```python
from build123d import *

# Parameters (mm, degrees)
PAD005_DEPTH    = 12
SKETCH025_R     = 2.5
POCKET019_DEPTH = 10
POCKET020_DEPTH = 1
SKETCH027_W     = 8
SKETCH027_H     = 8.3
POCKET021_DEPTH = 5
PAD006_DEPTH    = 3.5
SKETCH029_W     = 12.5
SKETCH029_H     = 5
POCKET022_DEPTH = 2


with BuildPart() as part:
    # Sketch024 → Pad005 (new body)
    with BuildSketch(Plane.XY):
        with BuildLine():
            ThreePointArc((0, 0), (0.0125001507, 3.6000868045), (0.05, 7.2))
            Line((0.05, 7.2), (0.75, 22.55))
            add(Edge.make_bspline(
                [(0.75, 22.55), (0.790433, 24.50555), (2.8995135699, 28.3383927733), (10.6468681476, 35.231617337), (14.5053016695, 34.8194742751), (20.1, 35.5)],
                knots=[0, 0, 0, 0, 0.3333333333, 0.6666666667, 1, 1, 1, 1], degree=3))
            Line((20.1, 35.5), (64.2, 35.5))
            add(Edge.make_bspline(
                [(92, 0), (92.391037, 11.810127), (88.126587, 35.076866), (64.2, 35.5)],
                knots=[0, 0, 0, 0, 1, 1, 1, 1], degree=3))
            Line((92, 0), (0, 0))
        make_face()
    extrude(amount=PAD005_DEPTH)

    # Sketch025 (on Face8 of Pad005) → Pocket019 (cut)
    with BuildSketch(Plane.XY.offset(12)):
        with Locations((17, 25)):
            Circle(SKETCH025_R)
        with BuildLine():
            ThreePointArc((84.5, 0), (82, 2.5), (79.5, 0))
            Line((79.5, 0), (84.5, 0))
        make_face()
        with BuildLine():
            Line((2, 0), (2.5758571429, 18.6857169977))
            ThreePointArc((7.6817324497, 29.5040514173), (4.0036624605, 24.625907301), (2.5758571429, 18.6857169977))
            ThreePointArc((11, 28), (9.8256709089, 29.8216112511), (7.6817324497, 29.5040514173))
            Line((11, 25), (11, 28))
            ThreePointArc((11, 25), (17, 19), (23, 25))
            Line((23, 25), (23, 31.5))
            ThreePointArc((25, 33.5), (23.5857864376, 32.9142135624), (23, 31.5))
            Line((25.1, 33.5), (25, 33.5))
            ThreePointArc((27.1, 31.5), (26.5142135624, 32.9142135624), (25.1, 33.5))
            Line((27.1, 12), (27.1, 31.5))
            ThreePointArc((27.1, 12), (27.6857864376, 10.5857864376), (29.1, 10))
            Line((31.1, 10), (29.1, 10))
            ThreePointArc((31.1, 10), (32.5142135624, 10.5857864376), (33.1, 12))
            Line((33.1, 31.5), (33.1, 12))
            ThreePointArc((35.1, 33.5), (33.6857864376, 32.9142135624), (33.1, 31.5))
            Line((49.3, 33.5), (35.1, 33.5))
            ThreePointArc((51.3, 31.5), (50.7142135624, 32.9142135624), (49.3, 33.5))
            Line((51.3, 12), (51.3, 31.5))
            ThreePointArc((51.3, 12), (51.8857864376, 10.5857864376), (53.3, 10))
            Line((55.3, 10), (53.3, 10))
            ThreePointArc((55.3, 10), (56.7142135624, 10.5857864376), (57.3, 12))
            Line((57.3, 31.4999999999), (57.3, 12))
            ThreePointArc((59.3, 33.4999999999), (57.8857864376, 32.9142135623), (57.3, 31.4999999999))
            Line((59.3, 33.5), (64.2, 33.5))
            ThreePointArc((87.491325765, 7.8139309331), (81.5019467421, 25.7859071373), (64.2, 33.5))
            ThreePointArc((85.5, 6), (86.8468225322, 6.521463877), (87.491325765, 7.8139309331))
            Line((82, 6), (85.5, 6))
            ThreePointArc((82, 6), (77.7573593129, 4.2426406871), (76, 0))
            Line((22, 0), (76, 0))
            Line((22, 1), (22, 0))
            Line((16, 1), (22, 1))
            Line((16, 0), (16, 1))
            Line((2, 0), (16, 0))
        make_face()
    extrude(amount=-POCKET019_DEPTH, mode=Mode.SUBTRACT)

    # Sketch026 (on Face3 of Pocket019) → Pocket020 (cut)
    with BuildSketch(Plane.XZ):
        Polygon((22, 12), (22, 4), (18, 10), (16, 10), (16, 12), align=None)
    extrude(amount=-POCKET020_DEPTH, mode=Mode.SUBTRACT)

    # Sketch027 → Pocket021 (cut)
    with BuildSketch(Plane.YZ):
        with Locations((4, 6.15)):
            Rectangle(SKETCH027_W, SKETCH027_H)
    extrude(amount=POCKET021_DEPTH, mode=Mode.SUBTRACT)

    # Sketch028 (on Face8 of Pocket021) → Pad006 (join)
    with BuildSketch(Plane.XY.offset(12)):
        with BuildLine():
            ThreePointArc((31.1, 10), (32.5142135624, 10.5857864376), (33.1, 12))
            Line((33.1, 12), (33.1, 14))
            ThreePointArc((33.1, 14), (32.5142135624, 15.4142135624), (31.1, 16))
            Line((29.1, 16), (31.1, 16))
            ThreePointArc((29.1, 16), (27.6857864376, 15.4142135624), (27.1, 14))
            Line((27.1, 12), (27.1, 14))
            ThreePointArc((27.1, 12), (27.6857864376, 10.5857864376), (29.1, 10))
            Line((29.1, 10), (31.1, 10))
        make_face()
        with BuildLine():
            ThreePointArc((51.3, 12), (51.8857864376, 10.5857864376), (53.3, 10))
            Line((53.3, 10), (55.3, 10))
            ThreePointArc((55.3, 10), (56.7142135624, 10.5857864376), (57.3, 12))
            Line((57.3, 12), (57.3, 14))
            ThreePointArc((57.3, 14), (56.7142135624, 15.4142135624), (55.3, 16))
            Line((53.3, 16), (55.3, 16))
            ThreePointArc((53.3, 16), (51.8857864376, 15.4142135624), (51.3, 14))
            Line((51.3, 12), (51.3, 14))
        make_face()
    extrude(amount=PAD006_DEPTH)

    # Mirrored002: part across XZ


with BuildPart() as part_1:
    add(part.part)
    add(part.part.mirror(Plane.XZ))

    # Sketch029 (on Face33 of Mirrored002) → Pocket022 (cut)
    with BuildSketch(Plane(origin=(0, 35.5, 0), x_dir=(-1, 0, 0), z_dir=(0, 1, 0))):
        with Locations((-42.65, 7)):
            Rectangle(SKETCH029_W, SKETCH029_H)
    extrude(amount=-POCKET022_DEPTH, mode=Mode.SUBTRACT)


with BuildPart() as part_2:
    # Body004 placement: moved
    add(part_1.part.moved(Location((0, 0, -12))))


solid = part_2.part
```
Verification items for the finished model (mm, model axes). A direction names the side the tool comes from. Round coordinates to 2 decimals unless told otherwise and drop trailing zeros. Answer as a JSON object with one key per item and string values. Group by question number.
Q1. Tool access check on faces 5 (the flat face through (18, -1, -7)), 6 (the cylindrical face through (32.53, -15.4, 1.73)), 7 (the flat face through (82, 0, -10)). Record the directions out of +Z, -Z, +X, -X, +Y, -Y that give a thin tool (end or side, any length) a straight path to the whole face; none if there is none.
Q2. Go/stop test with flat-tipped pins: pin 1 Ø3 at (y, z) = (12.5, -2) entering from -X; pin 2 Ø4 at (x, y) = (81, 13) entering from +Z; pin 3 Ø21.5 at (x, y) = (36, -4) entering from +Z; pin 4 Ø7 at (y, z) = (-17.5, -3) entering from +X. Record where each tip stops, or that it passes through.
Q3. Mould release check, pull along Y, two halves, no side actions. Record for faces 1 (the flat face through (54, 10, -3)), 2 (the cylindrical face through (32.5, -10.57, -3.34)), 3 (the flat face through (54, -13, 3.5)), 4 (the cylindrical face through (32.53, 15.4, 1.73)): released by +Y, released by -Y, zero draft, split by the parting line, or undercut.
Q4. Thickness scan on line 1 (Y direction, x = 84, z = -7.25); line 2 (X direction, y = -25, z = -5.5); line 3 (X direction, y = -12.5, z = -2.25). Record the ranges inside material, lowest first.
Q5. Section check A-A, the plane z = 1.5. Give the number of separate pieces and of enclosed holes in the cut face, plus the area to 3 significant figures.
Found:
{
 "1": {"face 5": "+Z, -X", "face 6": "+Z, -Y", "face 7": "+Z"},
 "2": {"pin 1": "stops at x = 0.22", "pin 2": "stops at z = -10", "pin 3": "stops at z = 3.5", "pin 4": "stops at x = 90.38"},
 "3": {"face 1": "undercut", "face 2": "undercut", "face 3": "zero draft", "face 4": "released by +Y"},
 "4": {"line 1": "y = -26.75 to -22.49, -6 to -1.5, 1.5 to 6, 22.49 to 26.75", "line 2": "x = 1.31 to 4.19, 11 to 14.5, 19.5 to 23, 27.1 to 33.1, 51.3 to 57.3, 82.18 to 85.36", "line 3": "x = 0.29 to 2.39, 27.1 to 33.1, 51.3 to 57.3, 87.46 to 90.76"},
 "5": {"separate pieces": "4", "enclosed holes": "0", "area": "130 mm^2"}
}
